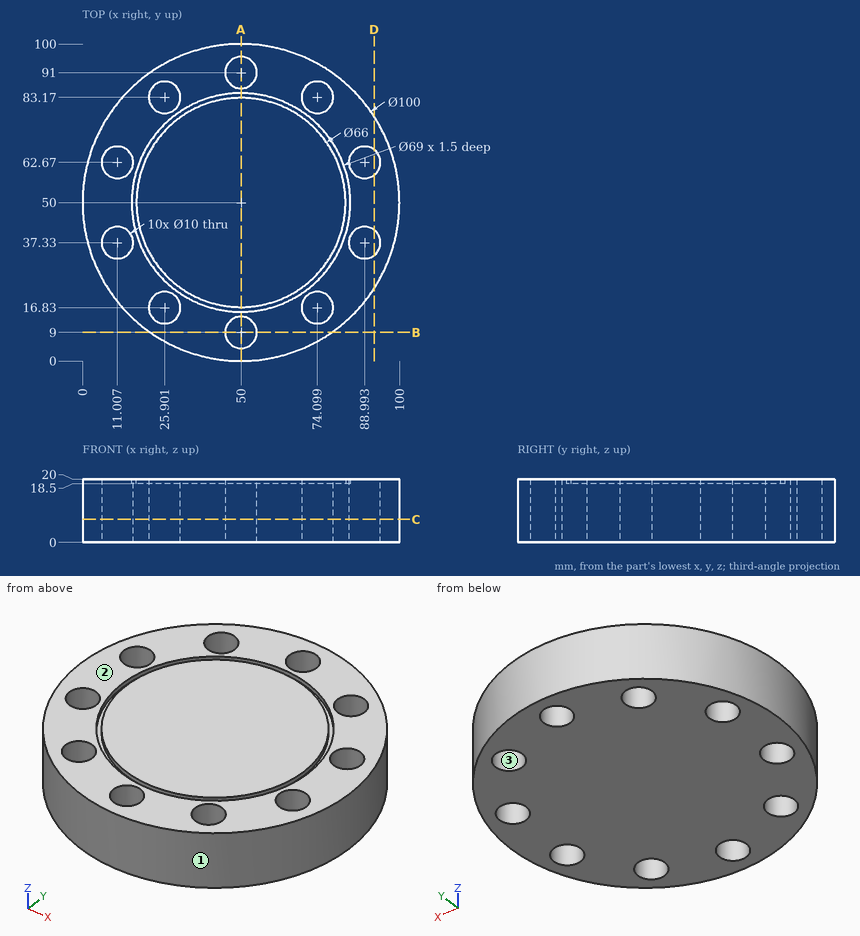
Check sheet for the drawn part. Datum: minimum x, y, z corner. Units: mm. Round coordinates to 2 decimals unless told otherwise and drop trailing zeros. Order: outer loops, then holes, each group sorted by start corner. A loop starts at its lowest first (then second) coordinate and runs counter-clockwise, first axis right, second up. Notation, with made-up numbers: M 51,-21 L 60,-21 A24 cw 60,-3 Z; hole C -27,16 d6. An arc over 180 degrees is marked long. Answer in a Markdown table with one row per item.
(1) Material ranges on line 1 along Y through (x, z) = (23.5, 8.5) (1 decimal); line 2 along Y through (x, z) = (11, 13.5); line 3 along X through (y, z) = (60, 9) (1 decimal), recorded low to high. Write a range as from..to.
Findings:
| item | result |
|---|---|
| line 1 | y = 7.6..12.4, 21.2..78.8, 87.6..92.4 |
| line 2 | y = 18.71..32.33, 42.33..57.67, 67.67..81.29 |
| line 3 | x = 1..6.8, 15.2..84.8, 93.2..99 |
(2) Draft check along X on the marked faces 1, 2 and 3. Enter one of: +X half, -X half, draft (parallel to the pull), parting line (faces both ways), or undercut.
Findings:
| item | result |
|---|---|
| face 1 | parting line |
| face 2 | draft |
| face 3 | undercut |
(3) Section check B-B on y = 9. Record the boundary of the cut face in (x, z).
Findings:
| item | result |
|---|---|
| outline | M 21.38,0 L 45,0 L 45,20 L 21.38,20 Z; M 55,0 L 78.62,0 L 78.62,20 L 55,20 Z |
(4) Section check C-C on z = 7.25. Give the number of separate pieces and of enclosed holes in the cut face, plus the area to 3 significant figures.
Findings:
| item | result |
|---|---|
| separate pieces | 1 |
| enclosed holes | 10 |
| area | 7,070 mm^2 |
(5) Gauge pin test, flat ends, axial feed: pin 1 (5 mm diameter, centred on x = 69, z = 12, fed in from +Y); pin 2 (2 mm diameter, centred on x = 63, z = 12.5, fed in from -Y); pin 3 (12 mm diameter, centred on x = 54.5, z = 17.5, fed in from +Y). Record the tip position at first contact, or that the pin passes through.
Findings:
| item | result |
|---|---|
| pin 1 | stops at y = 97.2 |
| pin 2 | stops at y = 1.46 |
| pin 3 | stops at y = 100 |
(6) Section check A-A on x = 50. Record the boundary of the cut face in (y, z).
Findings:
| item | result |
|---|---|
| outline | M 0,0 L 4,0 L 4,20 L 0,20 Z; M 14,0 L 86,0 L 86,20 L 84.5,20 L 84.5,18.5 L 83,18.5 L 83,20 L 17,20 L 17,18.5 L 15.5,18.5 L 15.5,20 L 14,20 Z; M 96,0 L 100,0 L 100,20 L 96,20 Z |
(7) Section check D-D on x = 92. Record the boundary of the cut face in (y, z) (1 decimal).
Findings:
| item | result |
|---|---|
| outline | M 22.9,0 L 33.3,0 L 33.3,20 L 22.9,20 Z; M 41.3,0 L 58.7,0 L 58.7,20 L 41.3,20 Z; M 66.7,0 L 77.1,0 L 77.1,20 L 66.7,20 Z |
